from build123d import *

# Parameters (mm, degrees)
EXTRUDE_1_DEPTH      = 1
F_3_0MM_1_AT_2_COUNT = 2
F_3_0MM_1_AT_2_PITCH = 12
F_3_0MM_1_AT_3_COUNT = 2
F_3_0MM_1_AT_3_PITCH = 30
F_3_0MM_1_AT_4_COUNT = 2
F_3_0MM_1_AT_4_PITCH = 60
F_3_0MM_1_AT_5_COUNT = 2
F_3_0MM_1_AT_5_PITCH = 32.310988843
F_3_0MM_1_AT_6_COUNT = 2
F_3_0MM_1_AT_6_PITCH = 61.188234163
F_3_0MM_1_AT_7_COUNT = 2
F_3_0MM_1_AT_7_PITCH = 78.006409993
F_3_0MM_1_AT_8_COUNT = 2
F_3_0MM_1_AT_8_PITCH = 90.005555384


with BuildPart() as part:
    # 草图1 → 凸台-拉伸1 (new body)
    with BuildSketch(Plane(origin=(0, 0, 0), x_dir=(1, 0, 0), z_dir=(0, 1, 0))):
        Polygon((100, 10), (80, 0), (0, 0), (0, 20), (100, 20), align=None)
    extrude(amount=EXTRUDE_1_DEPTH)

    # 草图3 → Ø3.0mm 暗销孔1 (revolve, cut)
    with BuildSketch(Plane(origin=(5, 1, -16), x_dir=(0, 0, 1), z_dir=(1, 0, 0))):
        Polygon((0, 0), (0, 1), (1.5, 1), (1.5, 0.025), (1.525, 0), align=None)
    f_3_0mm_1 = revolve(axis=Axis((5, 7.35, -16), (0, -1, 0)), mode=Mode.SUBTRACT)

    # Ø3.0mm 暗销孔1 at 2: Ø3.0mm 暗销孔1 ×2
    with Locations(*[(0, 0, i * F_3_0MM_1_AT_2_PITCH) for i in range(1, F_3_0MM_1_AT_2_COUNT)]):
        add(f_3_0mm_1, mode=Mode.SUBTRACT)

    # Ø3.0mm 暗销孔1 at 3: Ø3.0mm 暗销孔1 ×2
    with Locations(*[(i * F_3_0MM_1_AT_3_PITCH, 0, 0) for i in range(1, F_3_0MM_1_AT_3_COUNT)]):
        add(f_3_0mm_1, mode=Mode.SUBTRACT)

    # Ø3.0mm 暗销孔1 at 4: Ø3.0mm 暗销孔1 ×2
    with Locations(*[(i * F_3_0MM_1_AT_4_PITCH, 0, 0) for i in range(1, F_3_0MM_1_AT_4_COUNT)]):
        add(f_3_0mm_1, mode=Mode.SUBTRACT)

    # Ø3.0mm 暗销孔1 at 5: Ø3.0mm 暗销孔1 ×2
    with Locations(*[Vector(0.9284766908852593, 0, 0.37139067635410383) * (i * F_3_0MM_1_AT_5_PITCH) for i in range(1, F_3_0MM_1_AT_5_COUNT)]):
        add(f_3_0mm_1, mode=Mode.SUBTRACT)

    # Ø3.0mm 暗销孔1 at 6: Ø3.0mm 暗销孔1 ×2
    with Locations(*[Vector(0.9805806756909202, 0, 0.19611613513818404) * (i * F_3_0MM_1_AT_6_PITCH) for i in range(1, F_3_0MM_1_AT_6_COUNT)]):
        add(f_3_0mm_1, mode=Mode.SUBTRACT)

    # Ø3.0mm 暗销孔1 at 7: Ø3.0mm 暗销孔1 ×2
    with Locations(*[Vector(0.9999178273551348, 0, 0.01281945932506583) * (i * F_3_0MM_1_AT_7_PITCH) for i in range(1, F_3_0MM_1_AT_7_COUNT)]):
        add(f_3_0mm_1, mode=Mode.SUBTRACT)

    # Ø3.0mm 暗销孔1 at 8: Ø3.0mm 暗销孔1 ×2
    with Locations(*[Vector(0.9999382773199424, 0, 0.011110425303554916) * (i * F_3_0MM_1_AT_8_PITCH) for i in range(1, F_3_0MM_1_AT_8_COUNT)]):
        add(f_3_0mm_1, mode=Mode.SUBTRACT)


solid = part.part
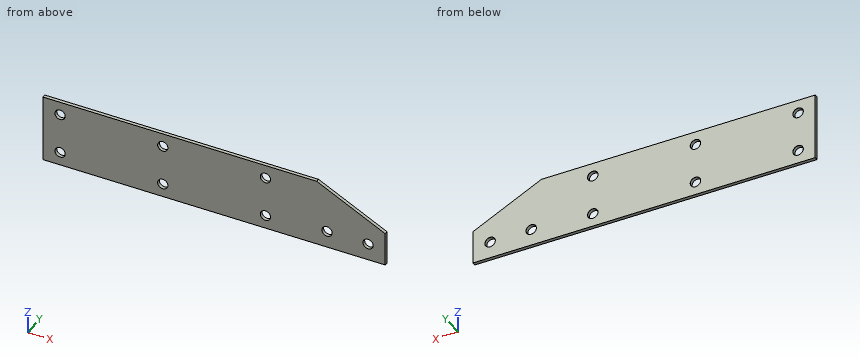
Geometry check sheet. Reference: the model listing, model coordinates, mm. Coordinates: 2 decimals unless noted, no trailing zeros. Write each loop counter-clockwise with the first axis right and the second up, starting at its lowest first coordinate (ties: lowest second). Pieces come first, ordered by that corner, then holes. Notation, with made-up numbers: (69, 18) -> (111, 18) arc R28 cw to (111, 52) -> close; hole circle Ø10 at (27, 33). An arc over 180 degrees is marked (long way). One line per question, with ' | ' between items.
1. Cross-section at D-D on z = -8.5. Record the cut outline in (x, y), and give its area (3 significant figures).
Answers:
outline: (0, 0) -> (97, 0) -> (97, 1) -> (0, 1) -> close | area: 97.0 mm²
2. Thickness scan on probe 1 along Z at (x, y) = (5, 0.25); probe 2 along X at (y, z) = (0.6, -2.75); probe 3 along X at (y, z) = (0.65, -13.75). Record the ranges inside material, lowest first. Write a range as from..to.
Answers:
probe 1: z = -20..-17.5, -14.5..-5.5, -2.5..0 | probe 2: x = 0..4.17, 5.83..34.17, 35.83..64.17, 65.83..85.5 | probe 3: x = 0..82.17, 83.83..94.17, 95.83..100
3. Depth check by flat-ended pin: pin 1 Ø2.5 at (x, z) = (83, -15) entering from +Y. Enter the tip coordinate at first touch or a pass-through.
Answers:
pin 1: passes through
4. Cross-section at B-B on x = 5. Record the cut outline in (y, z) (3 decimals), and give its area (3 significant figures).
Answers:
outline: (0, -20) -> (1, -20) -> (1, -17.525) -> (0.975, -17.5) -> (0, -17.5) -> close; (0, -14.5) -> (0.975, -14.5) -> (1, -14.475) -> (1, -5.525) -> (0.975, -5.5) -> (0, -5.5) -> close; (0, -2.5) -> (0.975, -2.5) -> (1, -2.475) -> (1, 0) -> (0, 0) -> close | area: 14.0 mm²
5. Cross-section at C-C on y = 0.45. State how many separate pieces and enclosed holes the cut face has, and give its area (3 significant figures).
Answers:
separate pieces: 1 | enclosed holes: 8 | area: 1,840 mm²
6. Cross-section at A-A on x = 83. Record the cut outline in (y, z) (3 decimals), and give its area (3 significant figures).
Answers:
outline: (0, -20) -> (1, -20) -> (1, -16.525) -> (0.975, -16.5) -> (0, -16.5) -> close; (0, -13.5) -> (0.975, -13.5) -> (1, -13.475) -> (1, -1.5) -> (0, -1.5) -> close | area: 15.5 mm²
